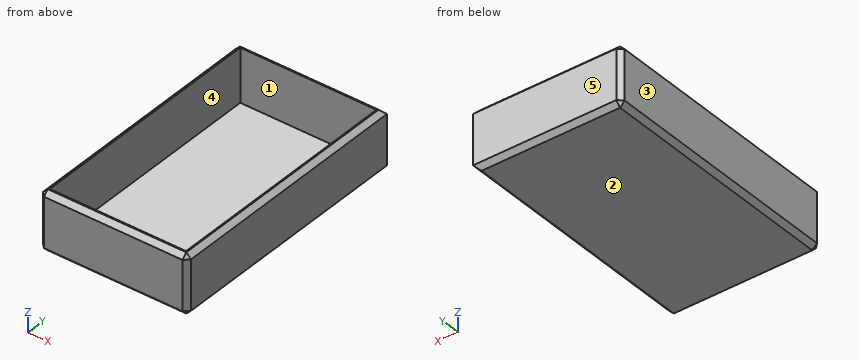
```python
from build123d import *

# Parameters (mm, degrees)
F0_W     = 62.507808
F0_H     = 107.542976
F1_DEPTH = 12.5
F2_T     = -2.5
F3_SIZE  = 2


with BuildPart() as f1:
    # F0 (on Top) → F1 (new body, symmetric)
    with BuildSketch(Plane.XY):
        Rectangle(F0_W, F0_H)
    extrude(amount=F1_DEPTH, both=True)

    # F2
    f2_openings = [f1.faces().sort_by_distance(p)[0] for p in [
        (0, 0, 12.5),
    ]]
    offset(amount=F2_T, openings=f2_openings)

    # F3
    f3_edges = [f1.edges().sort_by_distance(p)[0] for p in [
        (-31.253904, 53.771488, 0),
        (-31.253904, 0, -12.5),
        (-31.253904, 0, 12.5),
        (0, 53.771488, -12.5),
        (0, 53.771488, 12.5),
        (31.253904, 0, 12.5),
        (31.253904, 0, -12.5),
        (31.253904, -53.771488, 0),
        (0, -53.771488, -12.5),
        (0, -53.771488, 12.5),
        (-31.253904, -53.771488, 0),
    ]]
    chamfer(f3_edges, length=F3_SIZE)


solid = f1.part
```
Design review of the part built by this model. Coordinates are the model's own, in mm. Face numbers are marked on the shaded views. A direction names the side the tool comes from. Round coordinates to 2 decimals unless told otherwise and drop trailing zeros. Write each loop counter-clockwise with the first axis right and the second up, starting at its lowest first coordinate (ties: lowest second). Pieces come first, ordered by that corner, then holes.
Item 1: We need section A-A on x = -15. Write out the cut boundary in (y, z), and give its area (3 significant figures).
Item 2: We need section C-C on y = -23. Write out the cut boundary in (x, z), and give its area (3 significant figures).
Item 3: The part is to be moulded in two halves that separate along X. For the marked faces 3, 4 and 5, say which applies: +X half, -X half, draft (parallel to the pull), parting line (faces both ways), or undercut.
Item 4: Clearance check with a flat-ended pin moving along its axis: pin 1 Ø5 at (x, y) = (-3, 35.5) entering from +Z. State where the tip first meets the part, or that it passes through.
Item 5: For probe 1 along Y at (x, z) = (25, -0.25); probe 2 along X at (y, z) = (0.5, -0.25); probe 3 along Z at (x, y) = (21, 25), list the stretches that pass through material, from the lowest coordinate up.
Item 6: For the marked faces 1 and 2, list the 3-axis set-ups (+Z, -Z, +X, -X, +Y, -Y) from which the entire face can be reached by the end or side of a thin tool; tool diameter is ignored.
Item 7: We need section B-B on z = 3.5. Write out the cut boundary in (x, y), and give its area (3 significant figures).
Returned:
1. outline: (-53.77, -10.5) - (-51.77, -12.5) - (51.77, -12.5) - (53.77, -10.5) - (53.77, 10.5) - (51.77, 12.5) - (51.27, 12.5) - (51.27, -10) - (-51.27, -10) - (-51.27, 12.5) - (-51.77, 12.5) - (-53.77, 10.5) - close
1. area: 373 mm2
2. outline: (-31.25, -10.5) - (-29.25, -12.5) - (29.25, -12.5) - (31.25, -10.5) - (31.25, 10.5) - (29.25, 12.5) - (28.75, 12.5) - (28.75, -10) - (-28.75, -10) - (-28.75, 12.5) - (-29.25, 12.5) - (-31.25, 10.5) - close
2. area: 261 mm2
3. face 3: -X half
3. face 4: undercut
3. face 5: draft
4. pin 1: stops at z = -10
5. probe 1: y = -53.77 to -51.27, 51.27 to 53.77
5. probe 2: x = -31.25 to -28.75, 28.75 to 31.25
5. probe 3: z = -12.5 to -10
6. face 1: +Z
6. face 2: -Z, +X, -X, +Y, -Y
7. outline: (-31.25, -51.77) - (-29.25, -53.77) - (29.25, -53.77) - (31.25, -51.77) - (31.25, 53.77) - (-29.25, 53.77) - (-31.25, 51.77) - close; hole (-28.75, -51.27) - (28.75, -51.27) - (28.75, 51.27) - (-28.75, 51.27) - close
7. area: 819 mm2
